Autodesk Inventor part; units mm, degrees
ref_plane "YZ Plane" through (0, 0, 0) normal (1, 0, 0) x (0, 1, 0)
ref_plane "XZ Plane" through (0, 0, 0) normal (0, 1, 0) x (-1, 0, 0)
ref_plane "XY Plane" through (0, 0, 0) normal (0, 0, 1) x (1, 0, 0)
sketch "Sketch1" plane through (0, 0, 0) normal (0, 0, 1) x (1, 0, 0)
  circle A0 centre (0, 0) radius 1.15
  line L0 (0, 0) -> (18, 0) construction
  line L1 (0, -3) -> (18, -3)
  line L2 (18, 3) -> (0, 3)
  arc A1 (0, 3) -> (0, -3) centre (0, 0) ccw
  arc A2 (18, -3) -> (18, 3) centre (18, 0) ccw
  circle A3 centre (18, 0) radius 0.75
  point P0 (9, 0)
  dimension "d0" = 2.3
  dimension "d1" = 3
  dimension "d2" = 1.5
  dimension "d3" = 18
extrude "Extrusion1" add sketch "Sketch1" along normal blind 2
sketch "Sketch2" plane through (0, 0, 0) normal (0, 0, -1) x (-1, 0, 0)
  arc A0 (0, -3) -> (0, 3) centre (0, 0) ccw
  circle A1 centre (0, 0) radius 3
  circle A2 centre (0, 0) radius 1.15
  circle A3 centre (0, 0) radius 1.15
  point P0 (0, -3)
extrude "Extrusion2" add sketch "Sketch2" along normal blind 8
properties part number "ServoArm"
Here's how the part is built. I have some questions about the finished solid (model axes, mm). A direction names the side the tool comes from. Round coordinates to 2 decimals unless told otherwise and drop trailing zeros. Write each loop counter-clockwise with the first axis right and the second up, starting at its lowest first coordinate (ties: lowest second). Pieces come first, ordered by that corner, then holes.
Q1. If we section it at D-D on x = 9: Write out the boundary of the cut face in (y, z), plus the area to 3 significant figures.
Q2. Which directions (+Z, -Z, +X, -X, +Y, -Y) give clear straight access to the entire face, cutting with the end or side of a thin tool? Please do faces 5 (the flat face through (9, -3, 1)), 6 (the cylindrical face through (-3, 0, -3)).
Q3. If we section it at B-B on z = 1.75: Write out the boundary of the cut face in (x, y).
Q4. If we mould it in two halves opening along Y, with no side actions, what happens to faces 1 (the flat face through (9, 3, 1)), 2 (the cylindrical face through (21, 0, 1)), 3 (the cylindrical face through (17.405, 0.456, 0.986)), 4 (the flat face through (10, 0, 0))? For each: +Y half, -Y half, draft (parallel to the pull), parting line (faces both ways), or undercut.
Q5. Please list where these lines run through material, in increasing order: probe 1 along Y at (x, z) = (0, 0.8); probe 2 along Y at (x, z) = (18, 0.6); probe 3 along Z at (x, y) = (5.25, 2.15).
Q6. If we section it at C-C on x = 18.25: Write out the boundary of the cut face in (y, z).
Q7. Will these pins go through, and if not, where does the flat tip stop? P1, Ø1.8, axis at x = 14.5, y = -0.5, coming from the -Z side; P2, Ø2, axis at x = 18, y = 0, coming from the +Z side; P3, Ø2, axis at y = 2, z = -3.5, coming from the +X side.
Answer below:
1. outline: (-3, 0) - (3, 0) - (3, 2) - (-3, 2) - close
1. area: 12.0 mm2
2. face 5: +Z, -Z, +X, -X, -Y
2. face 6: -Z
3. outline: (0, -3) - (18, -3) arc R3 ccw to (18, 3) - (0, 3) arc R3 ccw to start; hole circle Ø2.3 at (0, 0); hole circle Ø1.5 at (18, 0)
4. face 1: +Y half
4. face 2: parting line
4. face 3: undercut
4. face 4: draft
5. probe 1: y = -3 to -1.15, 1.15 to 3
5. probe 2: y = -3 to -0.75, 0.75 to 3
5. probe 3: z = 0 to 2
6. outline: (-2.99, 0) - (-0.71, 0) - (-0.71, 2) - (-2.99, 2) - close; (0.71, 0) - (2.99, 0) - (2.99, 2) - (0.71, 2) - close
7. P1: stops at z = 0
7. P2: stops at z = 2
7. P3: stops at x = 2.83
